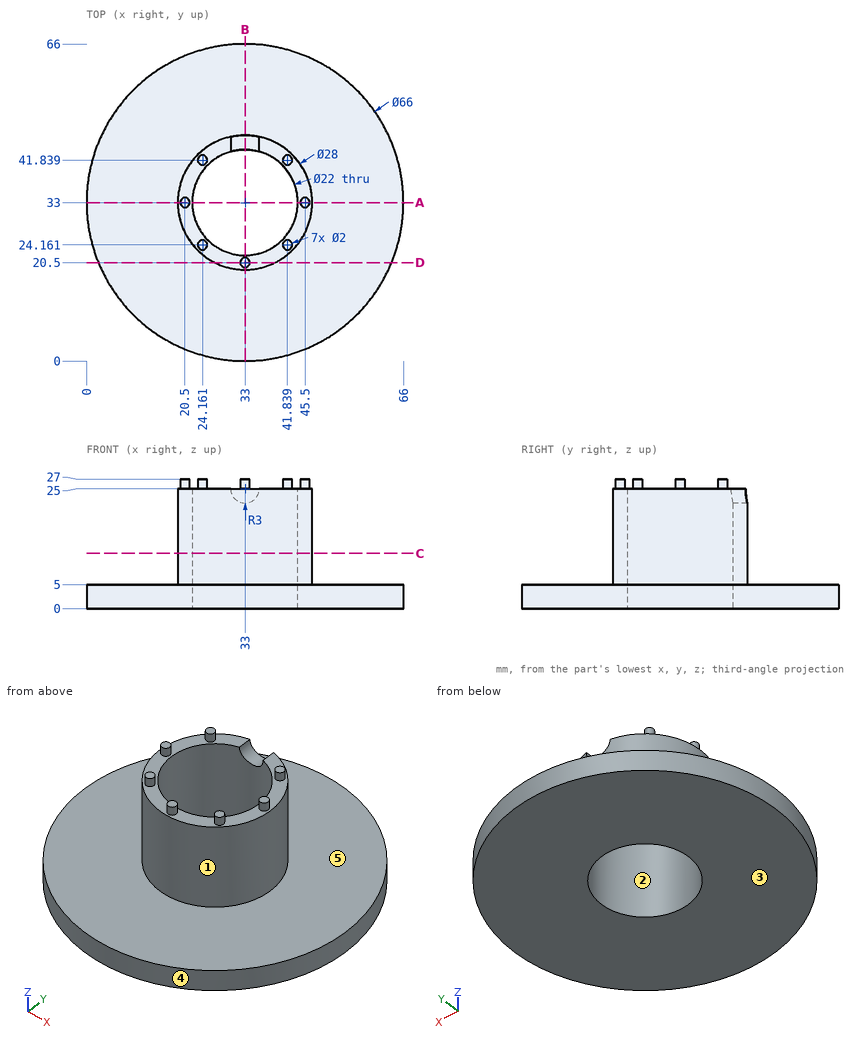
The drawing under review shows one solid part. Ordinate dimensions are in mm from its lowest x, y, z. A direction names the side the tool comes from. Round coordinates to 2 decimals unless told otherwise and drop trailing zeros. Loops run counter-clockwise (first coordinate to the right, second up) from the corner with the lowest first, then second, coordinate; pieces in that order, holes last. Notation, with made-up numbers: M 16,-13.5 L 42,-13.5 A13 ccw 42,-4.5 Z; hole C 16,-7 d5. An arc over 180 degrees is marked long. Answer as CSV lines item,"result". Start each with the question number.
Item 1: Wall thickness on line 1 (Y direction, x = 33, z = 6.5); line 2 (Z direction, x = 19, y = 54): over which ranges is each line inside the solid? List them lowest first. Write a range as [from, to].
Item 2: Consider section C-C (z = 11.5). Write out the cut boundary in (x, y), then the cut area to 3 significant figures.
Item 3: Consider section B-B (x = 33). Write out the cut boundary in (y, z).
Item 4: For the marked faces 4 and 5, list the 3-axis set-ups (+Z, -Z, +X, -X, +Y, -Y) from which the entire face can be reached by the end or side of a thin tool; tool diameter is ignored.
Item 5: Mouldability with a two-part tool opening along X and no side actions: class the marked faces 1, 2 and 3 as released by +X, released by -X, zero draft, split by the parting line, or undercut.
Item 6: Insertion check: P1, Ø20, axis at x = 33, y = 33, coming from the +Z side; P2, Ø10, axis at x = 15.5, z = 11, coming from the +Y side (1 decimal); P3, Ø6, axis at y = 18, z = 14.5, coming from the +X side; P4, Ø4, axis at x = 45, z = 4.5, coming from the -Y side. Each pin has a flat end and moves straight along its axis. Give the tip position at first contact, or say it passes through.
Item 7: Consider section D-D (y = 20.5). Write out the cut boundary in (x, z) (1 decimal).
Item 8: Consider section A-A (y = 33). Write out the cut boundary in (x, z).
Answer:
1,line 1,"y = [19, 22], [44, 47]"
1,line 2,"z = [0, 5]"
2,outline,"C 33,33 d28; hole C 33,33 d22"
2,area,"236 mm^2"
3,outline,"M 0,0 L 22,0 L 22,25 L 21.5,25 L 21.5,27 L 19.5,27 L 19.5,25 L 19,25 L 19,5 L 0,5 Z; M 44,0 L 66,0 L 66,5 L 47,5 L 47,22 L 44,22 Z"
4,face 4,"+Z, -Z"
4,face 5,"+Z"
5,face 1,"split by the parting line"
5,face 2,"undercut"
5,face 3,"zero draft"
6,P1,"passes through"
6,P2,"stops at y = 39.3"
6,P3,"stops at x = 40.21"
6,P4,"stops at y = 1.55"
7,outline,"M 2.5,0 L 63.5,0 L 63.5,5 L 39.3,5 L 39.3,25 L 34,25 L 34,27 L 32,27 L 32,25 L 26.7,25 L 26.7,5 L 2.5,5 Z"
8,outline,"M 0,0 L 22,0 L 22,25 L 21.5,25 L 21.5,27 L 19.5,27 L 19.5,25 L 19,25 L 19,5 L 0,5 Z; M 44,0 L 66,0 L 66,5 L 47,5 L 47,25 L 46.5,25 L 46.5,27 L 44.5,27 L 44.5,25 L 44,25 Z"
